For this review, take the finished solid that the model builds, in its own axes (mm). Give positions to 0.01 mm unless a question says otherwise; leave off trailing zeros. Order: outer loops, then holes, each group sorted by start corner. A loop starts at its lowest first (then second) coordinate and runs counter-clockwise, first axis right, second up. Notation, with made-up numbers: (19, 68) - (23, 68) arc R12 ccw to (23, 78) - close; hole circle Ø2 at (85.25, -11). An arc over 180 degrees is marked (long way). Use a Markdown table: item, result. Add a question column.
1) We need section A-A on y = 512.5. Write out the cut boundary in (x, z), then the cut area to 3 significant figures.
2) Wall thickness on L1, parallel to Y at x = 0, z = -11.6; L2, parallel to X at y = 983.5, z = -7; L3, parallel to Z at x = 12, y = 601.98: over which ranges is each line inside the solid? List them lowest first.
3) Clearance check with a flat-ended pin moving along its axis: P1, Ø2, axis at x = 0, y = 682.244, coming from the +Z side. State where the tip first meets the part, or that it passes through.
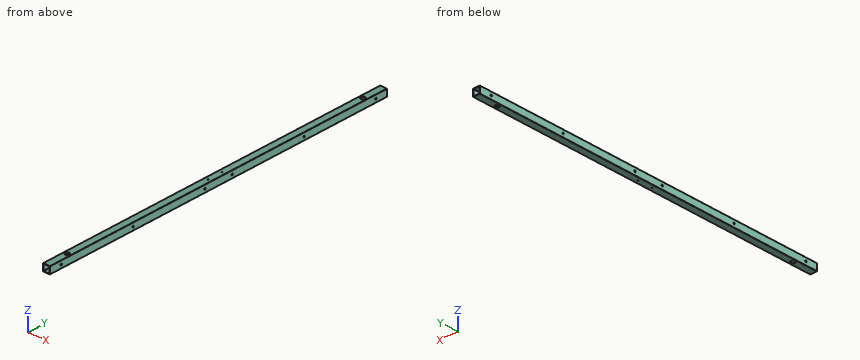
```python
from build123d import *

# Parameters (mm, degrees)
SKETCH1_W                        = 25.4
SKETCH1_H                        = 25.4
SKETCH1_W_2                      = 22.098
SKETCH1_H_2                      = 22.098
BOSS_EXTRUDE1_DEPTH              = 1309.624
FILLET1_R                        = 1.27
F_1_0_228_DIAMETER_HOLE1_D       = 5.7912
F_8_32_TAPPED_HOLE1_D            = 3.4544
F_39_64_0_60938_DIAMETER_HOLE1_D = 15.478252


with BuildPart() as part:
    # Sketch1 → Boss-Extrude1 (new body)
    with BuildSketch(Plane(origin=(0, 0, 0), x_dir=(1, 0, 0), z_dir=(0, 1, 0))):
        Rectangle(SKETCH1_W, SKETCH1_H)
        Rectangle(SKETCH1_W_2, SKETCH1_H_2, mode=Mode.SUBTRACT)
    extrude(amount=BOSS_EXTRUDE1_DEPTH)

    # Fillet1
    fillet1_edges = [part.edges().sort_by_distance(p)[0] for p in [
        (-11.049, 654.812, 11.049),
        (11.049, 654.812, 11.049),
        (11.049, 654.812, -11.049),
        (-11.049, 654.812, -11.049),
        (12.7, 654.812, 12.7),
        (-12.7, 654.812, 12.7),
        (-12.7, 654.812, -12.7),
        (12.7, 654.812, -12.7),
    ]]
    fillet(fillet1_edges, radius=FILLET1_R)

    # #1 (0.228) Diameter Hole1 (through all)
    with Locations(Plane(origin=(12.7, 0, 0), x_dir=(0, 0, -1), z_dir=(1, 0, 0))):
        with Locations((0, 601.98), (0, 1266.444), (0, 987.044), (0, 707.644), (0, 43.18), (0, 322.58)):
            Hole(F_1_0_228_DIAMETER_HOLE1_D / 2)

    # #8-32 Tapped Hole1 (through all)
    with Locations(Plane(origin=(0, 0, -12.7), x_dir=(-1, 0, 0), z_dir=(0, 0, -1))):
        with Locations((0, 627.38), (0, 682.244)):
            Hole(F_8_32_TAPPED_HOLE1_D / 2)

    # 39/64 (0.60938) Diameter Hole1 (through all)
    with Locations(Plane.XY.offset(12.7)):
        with Locations((0, 1229.36), (0, 80.264)):
            Hole(F_39_64_0_60938_DIAMETER_HOLE1_D / 2)


solid = part.part
```
Checked values:
| question | item | result |
|---|---|---|
| 1 | outline | (-12.7, -11.43) arc R1.27 ccw to (-11.43, -12.7) - (11.43, -12.7) arc R1.27 ccw to (12.7, -11.43) - (12.7, 11.43) arc R1.27 ccw to (11.43, 12.7) - (-11.43, 12.7) arc R1.27 ccw to (-12.7, 11.43) - close; hole (-11.05, -9.78) arc R1.27 ccw to (-9.78, -11.05) - (9.78, -11.05) arc R1.27 ccw to (11.05, -9.78) - (11.05, 9.78) arc R1.27 ccw to (9.78, 11.05) - (-9.78, 11.05) arc R1.27 ccw to (-11.05, 9.78) - close |
| 1 | area | 157 mm² |
| 2 | L1 | 0 to 72.52, 88 to 625.65, 629.11 to 680.52, 683.97 to 1221.62, 1237.1 to 1309.62 |
| 2 | L2 | -12.7 to -11.05, 11.05 to 12.7 |
| 2 | L3 | -12.56 to -2.9, 2.9 to 12.56 |
| 3 | P1 | through |
